from build123d import *

# Parameters (mm, degrees)
SKETCH_1_W             = 2
SKETCH_1_H             = 2
SM_BASE_FLANGE_1_DEPTH = 0.8
OTHER_START            = -3
OTHER_2_DEPTH          = 6
OTHER_START_2          = -1.75
OTHER_2_2_OUTLINE_W    = 0.8
OTHER_2_2_OUTLINE_H    = 1.5
OTHER_2_2_DEPTH        = 3.5
OTHER_2_3_DEPTH        = 6
OTHER_2_4_OUTLINE_W    = 0.8
OTHER_2_4_OUTLINE_H    = 2
OTHER_2_4_DEPTH        = 0.75
OTHER_START_3          = 1
OTHER_2_5_OUTLINE_W    = 0.8
OTHER_2_5_OUTLINE_H    = 2
OTHER_2_5_DEPTH        = 0.75
OTHER_2_6_DEPTH        = 0.8


with BuildPart() as part:
    # Базовая кромка1: sheet metal written as solids
    # Sketch 1 → Базовая кромка1 (new body)
    with BuildSketch(Plane(origin=(0, 0, 0), x_dir=(1, 0, 0), z_dir=(0, 1, 0))):
        Polygon((2.5, -1.75), (2.5, 1.75), (-1, 3), (-5, 3), (-5, 2.5), (-11.6, 2.5), (-12.6, 1.5), (-12.6, -1.5), (-11.6, -2.5), (-5, -2.5), (-5, -3), (-1, -3), align=None)
        with BuildLine():
            Line((-9.8875, 0.463512405), (-8.16875, 1.158781014))
            ThreePointArc((-8.16875, 1.158781014), (-6.45, 0), (-8.16875, -1.158781014))
            Line((-8.16875, -1.158781014), (-9.8875, -0.463512405))
            ThreePointArc((-9.8875, -0.463512405), (-10.2, 0), (-9.8875, 0.463512405))
        make_face(mode=Mode.SUBTRACT)
        Rectangle(SKETCH_1_W, SKETCH_1_H, mode=Mode.SUBTRACT)
    extrude(amount=-SM_BASE_FLANGE_1_DEPTH)

    # Other 2: read off the stored shape, not the designer's step
    # Other 2 outline → Other 2 (cut)
    with BuildSketch(Plane.XY.offset(OTHER_START)):
        with BuildLine():
            ThreePointArc((-2.299999999, 0), (-2.778889744, -0.581665383), (-3.5, -0.8))
            Line((-3.5, -0.8), (2.5, -0.8))
            Line((2.5, -0.8), (2.5, 0))
            Line((2.5, 0), (-2.299999999, 0))
        make_face()
    extrude(amount=OTHER_2_DEPTH, mode=Mode.SUBTRACT)

    # Other 2 2 outline → Other 2 2 (add)
    with BuildSketch(Plane.XY.offset(OTHER_START_2)):
        with Locations((-2.6, 4.336283306)):
            Rectangle(OTHER_2_2_OUTLINE_W, OTHER_2_2_OUTLINE_H)
        with BuildLine():
            Line((-2.2, 0.5), (-2.2, 1.586283306))
            Line((-2.2, 1.586283306), (-3, 1.586283306))
            Line((-3, 1.586283306), (-3, 0.5))
            ThreePointArc((-3, 0.5), (-3.146446609, 0.146446609), (-3.5, 0))
            Line((-3.5, 0), (-2.299999999, 0))
            ThreePointArc((-2.299999999, 0), (-2.225245121, 0.245049024), (-2.2, 0.5))
        make_face()
    extrude(amount=OTHER_2_2_DEPTH)

    # Other 2 3 outline → Other 2 3 (add)
    with BuildSketch(Plane.XY.offset(OTHER_START)):
        with BuildLine():
            Line((-2.2, 0.5), (-2.2, 1.586283306))
            Line((-2.2, 1.586283306), (-3, 1.586283306))
            Line((-3, 1.586283306), (-3, 0.5))
            ThreePointArc((-3, 0.5), (-3.146446609, 0.146446609), (-3.5, 0))
            Line((-3.5, 0), (-2.299999999, 0))
            ThreePointArc((-2.299999999, 0), (-2.225245121, 0.245049024), (-2.2, 0.5))
        make_face()
    extrude(amount=OTHER_2_3_DEPTH)

    # Other 2 4 outline → Other 2 4 (add)
    with BuildSketch(Plane.XY.offset(OTHER_START_2)):
        with Locations((-2.6, 2.586283306)):
            Rectangle(OTHER_2_4_OUTLINE_W, OTHER_2_4_OUTLINE_H)
    extrude(amount=OTHER_2_4_DEPTH)

    # Other 2 5 outline → Other 2 5 (add)
    with BuildSketch(Plane.XY.offset(OTHER_START_3)):
        with Locations((-2.6, 2.586283306)):
            Rectangle(OTHER_2_5_OUTLINE_W, OTHER_2_5_OUTLINE_H)
    extrude(amount=OTHER_2_5_DEPTH)

    # Other 2 6 outline → Other 2 6 (add)
    with BuildSketch(Plane.YZ.offset(OTHER_START)):
        Polygon((1.586283306, -1.75), (1.586283306, -3), (5.086283306, -1.75), align=None)
        Polygon((1.586283306, 1.75), (5.086283306, 1.75), (1.586283306, 3), align=None)
    extrude(amount=OTHER_2_6_DEPTH)


solid = part.part
Design review of the part built by this model. Coordinates are the model's own, in mm. A direction names the side the tool comes from. Give positions to 0.01 mm unless a question says otherwise; leave off trailing zeros. Order: outer loops, then holes, each group sorted by start corner. A loop starts at its lowest first (then second) coordinate and runs counter-clockwise, first axis right, second up. Notation, with made-up numbers: (-3, 35.25) - (14, 35.25) arc R29 ccw to (14, 55.25) - close; hole circle Ø7 at (75, 40.25). An arc over 180 degrees is marked (long way). Use CSV: the item, a comma, the result in double quotes. Start each with the question number.
Q1. Take a section at B-B (z = 0). State the section outline as (x, y) points, and give its area (3 significant figures).
Q2. For line 1 (Z direction, x = -7.7, y = -0.45); line 2 (Y direction, x = -10.75, z = 0.75); line 3 (X direction, y = 2.9, z = 2.45), list the stretches that pass through material, from the lowest coordinate up.
Q3. Machinability: for faces 1 (the face through (-3, 4, 0)), 2 (the face through (-2.2, 4, 0)), which of the approach directions +Z, -Z, +X, -X, +Y, -Y give a long, thin tool a straight path to every point of the face, cutting with its end or side? Answer none if there is none.
Q4. Take a section at D-D (z = -2.15). State the section outline as (x, y) points.
Q5. Take a section at A-A (x = -7.7). State the section outline as (y, z) points, and give its area (3 significant figures).
Q6. Draft analysis for pull direction Z (two halves, no side actions). For faces 3 (the face through (-8.1, 0, -1.4)), 4 (the face through (-12.1, -0.4, -2)), 5 (the face through (-12.1, -0.4, 2)), 6 (the face through (-6.45, -0.39, -0.03)), state which applies: pulls with the +Z half, pulls with the -Z half, needs draft (parallel to the pull), parting line crosses it, or undercut.
Q7. For P1, Ø0.6, axis at x = -8, y = -0.5, coming from the -Z side; P2, Ø1.4, axis at y = 2.5, z = 0.5, coming from the -X side; P3, Ø0.6, axis at x = -2.5, y = 2.5, coming from the +Z side; P4, Ø3, axis at x = -10, y = 2.5, coming from the +Z side, all flat-tipped, find the tip position at first contact; note any pin that passes through.
Q8. Take a section at C-C (y = 2.45). State the section outline as (x, z) points, and give its area (3 significant figures).
Calculated:
1,outline,"(-12.6, -0.8) - (-10.2, -0.8) - (-10.2, 0) - (-12.6, 0) - close; (-6.45, -0.8) - (-3.5, -0.8) arc R1.3 ccw to (-2.2, 0.5) - (-2.2, 1.59) - (-3, 1.59) - (-3, 0.5) arc R0.5 cw to (-3.5, 0) - (-6.45, 0) - close; (-3, 3.59) - (-2.2, 3.59) - (-2.2, 5.09) - (-3, 5.09) - close"
1,area,"7.48 mm²"
2,line 1,"z = -2.5 to -1.25, 1.25 to 2.5"
2,line 2,"y = -0.8 to 0"
2,line 3,"x = -3 to -2.2"
3,face 1,"+Z, -Z, -X, +Y"
3,face 2,"+Z, -Z, +X, +Y, -Y"
4,outline,"(-11.95, -0.8) - (-3.5, -0.8) arc R1.3 ccw to (-2.2, 0.5) - (-2.2, 3.97) - (-3, 3.97) - (-3, 0.5) arc R0.5 cw to (-3.5, 0) - (-11.95, 0) - close"
5,outline,"(-0.8, -2.5) - (0, -2.5) - (0, -1.25) - (-0.8, -1.25) - close; (-0.8, 1.25) - (0, 1.25) - (0, 2.5) - (-0.8, 2.5) - close"
5,area,"2.00 mm²"
6,face 3,"needs draft"
6,face 4,"pulls with the -Z half"
6,face 5,"pulls with the +Z half"
6,face 6,"undercut"
7,P1,"stops at z = -2.5"
7,P2,"stops at x = -3"
7,P3,"stops at z = 2.78"
7,P4,"passes through"
8,outline,"(-3, -2.69) - (-2.2, -2.69) - (-2.2, -1) - (-3, -1) - close; (-3, 1) - (-2.2, 1) - (-2.2, 2.69) - (-3, 2.69) - close"
8,area,"2.71 mm²"
